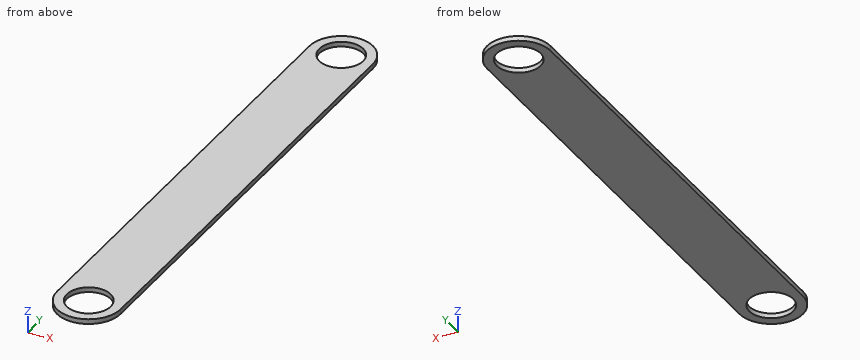
Autodesk Inventor part; units mm, degrees
ref_plane "YZ Plane" through (0, 0, 0) normal (1, 0, 0) x (0, 1, 0)
ref_plane "XZ Plane" through (0, 0, 0) normal (0, 1, 0) x (-1, 0, 0)
ref_plane "XY Plane" through (0, 0, 0) normal (0, 0, 1) x (1, 0, 0)
sketch "Sketch1" plane through (0, 0, 0) normal (0, 0, 1) x (1, 0, 0)
  arc A0 (-20.6375, 0) -> (20.6375, 0) centre (0, 0) ccw
  line L0 (-20.6375, 0) -> (-20.6375, 304.8)
  line L1 (20.6375, 0) -> (20.6375, 304.8)
  arc A1 (20.6375, 304.8) -> (-20.6375, 304.8) centre (0, 304.8) ccw
  circle A2 centre (0, 304.8) radius 14.2875
  circle A3 centre (0, 0) radius 14.2875
  arc A4 (-20.6375, 304.8) -> (20.6375, 304.8) centre (0, 304.8) ccw construction
  arc A5 (20.6375, 0) -> (-20.6375, 0) centre (0, 0) ccw construction
  dimension "d0" = 304.8
  dimension "d2" = 28.575
  dimension "d3" = 6.35
extrude "Extrusion1" add sketch "Sketch1" along normal blind 3.175
properties part number "upper-arm-panel"
Verification items for the finished model (mm, model axes). Round coordinates to 2 decimals unless told otherwise and drop trailing zeros. Write each loop counter-clockwise with the first axis right and the second up, starting at its lowest first coordinate (ties: lowest second). Pieces come first, ordered by that corner, then holes.
1. Section check B-B on z = 0.9. Enter the section's corners in (x, y) (1 decimal), plus the area to 3 significant figures.
2. Section check A-A on x = 0. Enter the section's corners in (y, z) (1 decimal).
3. Scan lines: L1, parallel to Y at x = 0, z = 1.1; L2, parallel to X at y = 303.5, z = 2.7; L3, parallel to Y at x = -12.5, z = 1. Record each from-to range of solid material in increasing order.
4. Gauge pin test, flat ends, axial feed: P1, Ø1.5, axis at x = 11.5, z = 3, coming from the -Y side; P2, Ø1.5, axis at x = -14.5, z = 0.5, coming from the -Y side. Record the tip position at first contact, or that the pin passes through.
Answer:
1. outline: (-20.6, 0) arc R20.6 ccw to (20.6, 0) - (20.6, 304.8) arc R20.6 ccw to (-20.6, 304.8) - close; hole circle Ø28.6 at (0, 0); hole circle Ø28.6 at (0, 304.8)
1. area: 12,600 mm2
2. outline: (-20.6, 0) - (-14.3, 0) - (-14.3, 3.2) - (-20.6, 3.2) - close; (14.3, 0) - (290.5, 0) - (290.5, 3.2) - (14.3, 3.2) - close; (319.1, 0) - (325.4, 0) - (325.4, 3.2) - (319.1, 3.2) - close
3. L1: y = -20.64 to -14.29, 14.29 to 290.51, 319.09 to 325.44
3. L2: x = -20.64 to -14.23, 14.23 to 20.64
3. L3: y = -16.42 to -6.92, 6.92 to 297.88, 311.72 to 321.22
4. P1: stops at y = -17.62
4. P2: stops at y = -15.39
